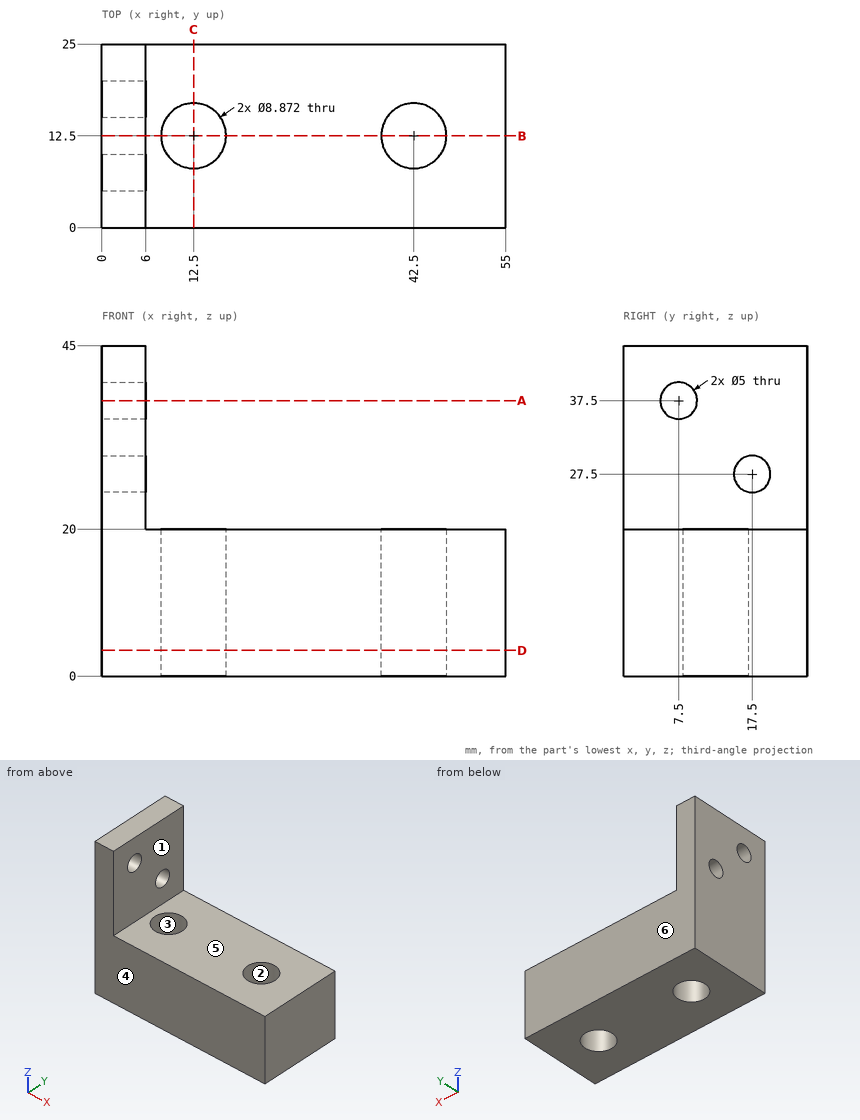
Part print with two shaded views. Sizes in mm from the minimum x, y, z corner. A direction names the side the tool comes from. Round coordinates to 2 decimals unless told otherwise and drop trailing zeros. Write each loop counter-clockwise with the first axis right and the second up, starting at its lowest first coordinate (ties: lowest second). Pieces come first, ordered by that corner, then holes. Notation, with made-up numbers: M 29.25,0 L 36.25,0 A16 cw 36.25,17 Z; hole C 5.25,39 d11. An arc over 180 degrees is marked long. Answer as CSV lines item,"result". Start each with the question number.
1) Band-saw the part on C-C (x = 12.5). List the corners of the cut face in (y, z), then the cut area to 3 significant figures.
2) Mould opens along Y. For the marked faces 1, 2, 3 and 4 say: +Y half, -Y half, draft (parallel to the pull), parting line (faces both ways), or undercut.
3) Which spindle directions (+Z, -Z, +X, -X, +Y, -Y) get a long thin tool onto all of the face, cutting with end or side? Do the marked faces 5 and 6. Say none if no direction does.
4) Band-saw the part on A-A (z = 37.5). List the corners of the cut face in (x, y), then the cut area to 3 significant figures.
5) Drill centre lines: L1, parallel to X at y = 13.5, z = 9; L2, parallel to Y at x = 2.95, z = 37.5; L3, parallel to Z at x = 23, y = 20. Where is each one in solid material? Low to high.
6) Drop flat-ended pins along their axis: pin 1 (12.5 mm diameter, centred on y = 18.5, z = 33.5, fed in from +X); pin 2 (8 mm diameter, centred on x = 45, y = 13.5, fed in from +Z); pin 3 (1 mm diameter, centred on x = 28.5, z = 21.5, fed in from -Y). Give the stop position or say it passes through.
7) Band-saw the part on D-D (z = 3.5). List the corners of the cut face in (x, y).
8) Band-saw the part on B-B (y = 12.5). List the corners of the cut face in (x, z), then the cut area to 3 significant figures.
Worked out:
1,outline,"M 0,0 L 8.06,0 L 8.06,20 L 0,20 Z; M 16.94,0 L 25,0 L 25,20 L 16.94,20 Z"
1,area,"323 mm²"
2,face 1,"draft"
2,face 2,"undercut"
2,face 3,"undercut"
2,face 4,"-Y half"
3,face 5,"+Z, +X, +Y, -Y"
3,face 6,"+Z, -Z, +X, -X, +Y"
4,outline,"M 0,0 L 6,0 L 6,5 L 0,5 Z; M 0,10 L 6,10 L 6,25 L 0,25 Z"
4,area,"120 mm²"
5,L1,"0 to 8.18, 16.82 to 38.18, 46.82 to 55"
5,L2,"0 to 5, 10 to 25"
5,L3,"0 to 20"
6,pin 1,"x = 6"
6,pin 2,"z = 20"
6,pin 3,"through"
7,outline,"M 0,0 L 55,0 L 55,25 L 0,25 Z; hole C 12.5,12.5 d8.87; hole C 42.5,12.5 d8.87"
8,outline,"M 0,0 L 8.06,0 L 8.06,20 L 6,20 L 6,45 L 0,45 Z; M 16.94,0 L 38.06,0 L 38.06,20 L 16.94,20 Z; M 46.94,0 L 55,0 L 55,20 L 46.94,20 Z"
8,area,"895 mm²"
